The listing builds one solid part. Answer for the finished solid, in the listing's coordinates (mm). Round coordinates to 2 decimals unless told otherwise and drop trailing zeros. Loops run counter-clockwise (first coordinate to the right, second up) from the corner with the lowest first, then second, coordinate; pieces in that order, holes last. Notation, with made-up numbers: (-13.75, 56.5) -> (30.25, 56.5) arc R19 cw to (30.25, 62.5) -> close; hole circle Ø9 at (-5.5, -2.5). An arc over 180 degrees is marked (long way). One line per question, with ' | ' between items.
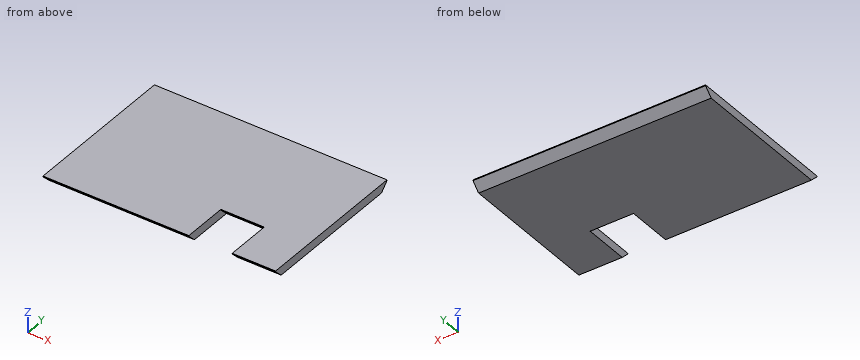
from build123d import *

# Parameters (mm, degrees)
F1_DEPTH = 2.2
F2_SIZE  = 2
F3_SIZE  = 2


with BuildPart() as f1:
    # F0 (on Top) → F1 (new body)
    with BuildSketch(Plane.XY):
        Polygon((-0.1190041415, 38.1740419386), (-59.1190041415, 38.1740419386), (-59.1190041415, -1.8259580614), (-22.1190041415, -1.8259580614), (-22.1190041415, 9.6740419386), (-11.1190041415, 9.6740419386), (-11.1190041415, -1.8259580614), (-0.1190041415, -1.8259580614), align=None)
    extrude(amount=F1_DEPTH)

    # F2
    f2_edges = [f1.edges().sort_by_distance(p)[0] for p in [
        (-29.619004, 38.174042, 0),
        (-40.619004, -1.825958, 0),
    ]]
    chamfer(f2_edges, length=F2_SIZE)

    # F3
    f3_edges = [f1.edges().sort_by_distance(p)[0] for p in [
        (-16.619004, 9.674042, 0),
        (-5.619004, -1.825958, 0),
    ]]
    chamfer(f3_edges, length=F3_SIZE)


solid = f1.part
Q1. A cutting plane is placed at A-A on y = 1.5. Give the vertices of the cut face in (x, z).
Numbers:
outline: (-59.12, 0) -> (-22.12, 0) -> (-22.12, 2.2) -> (-59.12, 2.2) -> close; (-11.12, 0) -> (-0.12, 0) -> (-0.12, 2.2) -> (-11.12, 2.2) -> close
Q2. A cutting plane is placed at B-B on x = -13.5. Give the vertices of the cut face in (y, z).
Numbers:
outline: (9.67, 2) -> (11.67, 0) -> (36.17, 0) -> (38.17, 2) -> (38.17, 2.2) -> (9.67, 2.2) -> close
Q3. A cutting plane is placed at C-C on z = 1.35. Give the vertices of the cut face in (x, y).
Numbers:
outline: (-59.12, -1.18) -> (-22.12, -1.18) -> (-22.12, 10.32) -> (-11.12, 10.32) -> (-11.12, -1.18) -> (-0.12, -1.18) -> (-0.12, 37.52) -> (-59.12, 37.52) -> close
Q4. Find the intervals of material crossed by line 1 (X direction, y = 10, z = 1); line 2 (Y direction, x = -4, z = 1.45); line 3 (Y direction, x = -5.5, z = 1.1), in increasing order. Write a range as from..to.
Numbers:
line 1: -59.12..-22.12, -11.12..-0.12 | line 2: -1.28..37.62 | line 3: -0.93..37.27
